Part model, mm, in its own coordinate system. Face numbers are marked on the shaded views. A direction names the side the tool comes from. Give positions to 0.01 mm unless a question says otherwise; leave off trailing zeros. Order: outer loops, then holes, each group sorted by start corner. A loop starts at its lowest first (then second) coordinate and runs counter-clockwise, first axis right, second up. Notation, with made-up numbers: (51, 7.5) - (103, 7.5) arc R16 ccw to (103, 34.5) - close; hole circle Ø3 at (80.5, 31). An arc over 180 degrees is marked (long way). One line per item, written item: value.
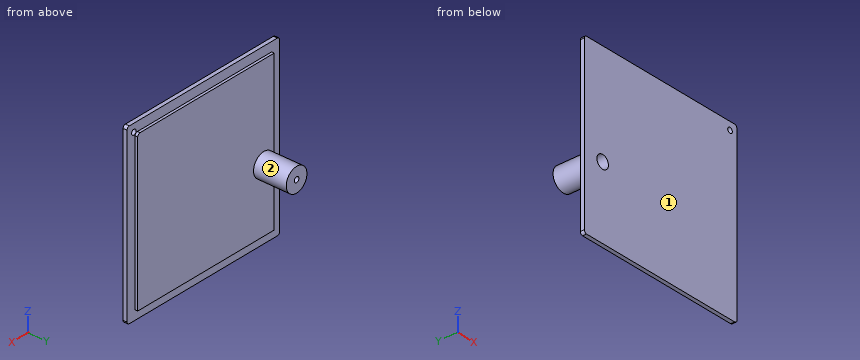
Autodesk Inventor part; units mm, degrees
ref_plane "YZ Plane" through (0, 0, 0) normal (1, 0, 0) x (0, 1, 0)
ref_plane "XZ Plane" through (0, 0, 0) normal (0, 1, 0) x (-1, 0, 0)
ref_plane "XY Plane" through (0, 0, 0) normal (0, 0, 1) x (1, 0, 0)
sketch "Esboço1" plane through (0, 0, 0) normal (0, 1, 0) x (-1, 0, 0)
  line L0 (-66.5, 66.5) -> (66.5, 66.5)
  line L1 (66.5, 66.5) -> (66.5, -66.5)
  line L2 (66.5, -66.5) -> (-66.5, -66.5)
  line L3 (-66.5, -66.5) -> (-66.5, 66.5)
  line L4 (-66.5, 66.5) -> (66.5, -66.5) construction
  line L5 (66.5, 66.5) -> (-66.5, -66.5) construction
  point P0 (0, 0)
  dimension "d0" = 133
  dimension "d1" = 133
extrude "Extrusão1" add sketch "Esboço1" along normal blind 3
sketch "Esboço2" plane through (0, 3, 0) normal (0, 1, 0) x (1, 0, 0)
  line L0 (59.5, -59.5) -> (-59.5, -59.5)
  line L1 (-59.5, -59.5) -> (-59.5, 59.5)
  line L2 (-59.5, 59.5) -> (59.5, 59.5)
  line L3 (59.5, 59.5) -> (59.5, -59.5)
  line L4 (59.5, -59.5) -> (-59.5, 59.5) construction
  line L5 (-59.5, -59.5) -> (59.5, 59.5) construction
  line L6 (-66.5, 66.5) -> (-66.5, -66.5)
  line L7 (66.5, 66.5) -> (-66.5, 66.5)
  point P0 (0, 0)
  dimension "d4" = 7
  dimension "d5" = 7
extrude "Extrusão2" add sketch "Esboço2" along normal blind 2
sketch "Esboço3" plane through (0, 5, 0) normal (0, 1, 0) x (1, 0, 0)
  circle A0 centre (-50.5, 11.5) radius 9
  line L0 (-66.5, -66.5) -> (66.5, -66.5)
  line L1 (-66.5, 66.5) -> (-66.5, -66.5)
  line L2 (66.5, 66.5) -> (-66.5, 66.5)
  point P0 (0, 0)
  dimension "d8" = 18
  dimension "d10" = 16
  dimension "d20" = 55
extrude "Extrusão3" add sketch "Esboço3" along normal blind 25
sketch "Esboço4" plane through (0, 0, 0) normal (0, -1, 0) x (1, 0, 0)
  circle A0 centre (-50.5, -11.5) radius 9
  circle A1 centre (-50.5, -11.5) radius 2
  point P0 (0, 0)
  dimension "d13" = 4
extrude "Extrusão4" cut sketch "Esboço4" against normal blind 31.25 contours A1
sketch "Esboço5" plane through (0, 0, 0) normal (0, -1, 0) x (1, 0, 0)
  circle A0 centre (-50.5, -11.5) radius 2
  circle A1 centre (-50.5, -11.5) radius 5
  point P0 (0, 0)
  dimension "d16" = 10
extrude "Extrusão5" cut sketch "Esboço5" against normal blind 24
fillet "Arredondamento1" radius 2 4 edges at (-66.5, 1.5, -66.5) (66.5, 1.5, -66.5) (66.5, 1.5, 66.5) (-66.5, 1.5, 66.5)
sketch "Esboço6" plane through (0, 0, 0) normal (0, -1, 0) x (1, 0, 0)
  circle A0 centre (60.5, 60.5) radius 2
  line L0 (-64.5, 66.5) -> (64.5, 66.5)
  line L1 (66.5, 64.5) -> (66.5, -64.5)
  point P0 (0, 0)
  dimension "d21" = 4
  dimension "d22" = 6
  dimension "d23" = 6
fillet "Arredondamento2" radius 2 1 edges at (59.5, 4, 59.5)
extrude "Extrusão6" cut sketch "Esboço6" against normal blind 10
properties part number "tampa caixa armazenamneto"
1) Wall check: line 1 along Z through (x, y) = (60.5, 2.3); line 2 along Z through (x, y) = (-50.5, 14.75); line 3 along Y through (x, z) = (7, -32). Give the ranges that are in metal, low to high. Write a range as [from, to].
Answer:
line 1: z = [-66.5, 58.5], [62.5, 66.5]
line 2: z = [-20.5, -16.5], [-6.5, -2.5]
line 3: y = [0, 5]
2) Drop flat-ended pins along their axis: P1, Ø5, axis at x = -20.5, z = 33.5, coming from the -Y side; P2, Ø0.6, axis at y = 3.5, z = -18.5, coming from the -X side; P3, Ø1.6, axis at y = 4.5, z = 17.5, coming from the +X side; P4, Ø3, axis at x = -53, z = -13, coming from the -Y side. Give the stop position or say it passes through.
Answer:
P1: stops at y = 0
P2: stops at x = -59.5
P3: stops at x = 59.5
P4: stops at y = 24
3) Slice it at C-C on x = -32. Write the cut outline in (y, z), then the cut area to 3 significant figures.
Answer:
outline: (0, -66.5) - (3, -66.5) - (3, -59.5) - (5, -59.5) - (5, 59.5) - (3, 59.5) - (3, 66.5) - (0, 66.5) - close
area: 637 mm2
4) Slice it at A-A on x = -50.5. Write the cut outline in (y, z), then the cut area to 3 significant figures.
Answer:
outline: (0, -66.5) - (3, -66.5) - (3, -59.5) - (5, -59.5) - (5, -20.5) - (30, -20.5) - (30, -13.5) - (24, -13.5) - (24, -16.5) - (0, -16.5) - close; (0, -6.5) - (24, -6.5) - (24, -9.5) - (30, -9.5) - (30, -2.5) - (5, -2.5) - (5, 59.5) - (3, 59.5) - (3, 66.5) - (0, 66.5) - close
area: 823 mm2
5) Which spindle directions (+Z, -Z, +X, -X, +Y, -Y) get a long thin tool onto all of the face, cutting with end or side? Do the marked faces 1 and 2. Say none if no direction does.
Answer:
face 1: +Z, -Z, +X, -X, -Y
face 2: +Y
6) Slice it at D-D on y = 17. Write the cut outline in (x, z), then the cut area to 3 significant figures.
Answer:
outline: circle Ø18 at (-50.5, -11.5); hole circle Ø10 at (-50.5, -11.5)
area: 176 mm2
7) Slice it at B-B on z = -48.5. Write the cut outline in (x, y), then the cut area to 3 significant figures.
Answer:
outline: (-66.5, 0) - (66.5, 0) - (66.5, 3) - (59.5, 3) - (59.5, 5) - (-59.5, 5) - (-59.5, 3) - (-66.5, 3) - close
area: 637 mm2
